Geometry: final body of the model. Coordinates: model frame, mm. Face numbers are marked on the shaded views. A direction names the side the tool comes from. Give positions to 0.01 mm unless a question says otherwise; leave off trailing zeros. Write each loop counter-clockwise with the first axis right and the second up, starting at its lowest first coordinate (ties: lowest second). Pieces come first, ordered by that corner, then holes. Notation, with made-up numbers: (-5, 67) -> (15, 67) arc R28 cw to (15, 86) -> close; hole circle Ø11 at (-20, 48). An arc over 180 degrees is marked (long way). Use CSV: the item, a comma, the result in double quotes. Start each with the question number.
1) Draft query along X for the marked faces 1, 2, 3 and 4. Return one class per face: pulls with the +X half, pulls with the -X half, needs draft (parallel to the pull), parting line crosses it, or undercut.
2) Material intervals for line 1 (Y direction, x = -26, z = 1.9); line 2 (X direction, y = 15.5, z = 6.25); line 3 (Z direction, x = -39, y = -1.5), sorted ascending. Write a range as [from, to].
3) Section D-D (y = -1). Output: boundary loops of the cut face in (x, z).
4) Set-up query: the marked faces 5, 6 and 7. Return all of +Z, -Z, +X, -X, +Y, -Y with unobstructed straight access to the full face (end or side cutting, diameter ignored); none if empty.
5) Contact query for flat-ended pins moving along their axis: P1, Ø3, axis at x = 29, z = 17.5, coming from the +Y side; P2, Ø7, axis at x = 7, y = -15.5, coming from the +Z side; P3, Ø21, axis at x = -44, y = -10.5, coming from the -Z side; P4, Ø2, axis at x = -37, y = 12, coming from the +Z side. Output: stop coordinate, or through.
6) Section C-C (y = -46). Output: boundary loops of the cut face in (x, z).
7) Section B-B (z = 11.25). Output: boundary loops of the cut face in (x, y), plus the area to 3 significant figures.
8) Section A-A (x = -26). Output: boundary loops of the cut face in (y, z), plus the area to 3 significant figures.
```python
from build123d import *

# Parameters (mm, degrees)
CROQUIS1_W              = 116
CROQUIS1_H              = 112
SALIENTE_EXTRUIR1_DEPTH = 3
CROQUIS2_W              = 24
CROQUIS2_H              = 48
SALIENTE_EXTRUIR2_DEPTH = 16
CROQUIS3_W              = 32
CROQUIS3_H              = 17
SALIENTE_EXTRUIR3_DEPTH = 22
VACIADO1_START          = -21.5
VACIADO1_OUTLINE_W      = 27
VACIADO1_OUTLINE_H      = 22.5
VACIADO1_OUTLINE_W_2    = 19
VACIADO1_OUTLINE_H_2    = 14
VACIADO1_DEPTH          = 14.5
VACIADO1_START_2        = -7
VACIADO1_2_OUTLINE_W    = 19
VACIADO1_2_OUTLINE_H    = 14
VACIADO1_2_DEPTH        = 28.5
CROQUIS5_W              = 27
CROQUIS5_H              = 2.5
SALIENTE_EXTRUIR7_DEPTH = 14.5
CORTAR_EXTRUIR1_DEPTH   = 34.5
CROQUIS7_R              = 1.5
CORTAR_EXTRUIR2_DEPTH   = 34.5


# Read off the part's stored shape, not the designer's step: Vaciado1
with BuildPart() as part:
    # Croquis1 → Saliente-Extruir1 (new body)
    with BuildSketch(Plane.XY):
        Rectangle(CROQUIS1_W, CROQUIS1_H)
    extrude(amount=SALIENTE_EXTRUIR1_DEPTH)

    # Croquis2 → Saliente-Extruir2 (add)
    with BuildSketch(Plane.XY.offset(3)):
        with Locations((-40, 0)):
            Rectangle(CROQUIS2_W, CROQUIS2_H)
    extrude(amount=SALIENTE_EXTRUIR2_DEPTH)

    # Croquis3 → Saliente-Extruir3 (add)
    with BuildSketch(Plane.XY.offset(3)):
        with Locations((10, -15.5)):
            Rectangle(CROQUIS3_W, CROQUIS3_H)
    extrude(amount=SALIENTE_EXTRUIR3_DEPTH)

    # Vaciado1 outline → Vaciado1 (cut)
    with BuildSketch(Plane(origin=(0, 0, 0), x_dir=(1, 0, 0), z_dir=(0, 1, 0)).offset(VACIADO1_START)):
        with Locations((10, -13.75)):
            Rectangle(VACIADO1_OUTLINE_W, VACIADO1_OUTLINE_H)
        with Locations((-40, -9.5)):
            Rectangle(VACIADO1_OUTLINE_W_2, VACIADO1_OUTLINE_H_2)
    extrude(amount=VACIADO1_DEPTH, mode=Mode.SUBTRACT)

    # Vaciado1 2 outline → Vaciado1 2 (cut)
    with BuildSketch(Plane(origin=(0, 0, 0), x_dir=(1, 0, 0), z_dir=(0, 1, 0)).offset(VACIADO1_START_2)):
        with Locations((-40, -9.5)):
            Rectangle(VACIADO1_2_OUTLINE_W, VACIADO1_2_OUTLINE_H)
    extrude(amount=VACIADO1_2_DEPTH, mode=Mode.SUBTRACT)

    # Croquis5 → Saliente-Extruir7 (add)
    with BuildSketch(Plane(origin=(0, -21.5, 0), x_dir=(1, 0, 0), z_dir=(0, 1, 0))):
        with Locations((10, -3.75)):
            Rectangle(CROQUIS5_W, CROQUIS5_H)
    extrude(amount=SALIENTE_EXTRUIR7_DEPTH)

    # Croquis6 → Cortar-Extruir1 (cut)
    with BuildSketch(Plane(origin=(26, 0, 0), x_dir=(0, 0, -1), z_dir=(1, 0, 0))):
        Polygon((-25, -7), (-25, -21.5), (-5.5, -7), align=None)
    extrude(amount=-CORTAR_EXTRUIR1_DEPTH, mode=Mode.SUBTRACT)

    # Croquis7 → Cortar-Extruir2 (cut)
    with BuildSketch(Plane.XY.offset(3)):
        with Locations((-26, 46)):
            Circle(CROQUIS7_R)
        with Locations((46, 46)):
            Circle(CROQUIS7_R)
        with Locations((0, -46)):
            Circle(CROQUIS7_R)
    extrude(amount=-CORTAR_EXTRUIR2_DEPTH, mode=Mode.SUBTRACT)


solid = part.part
```
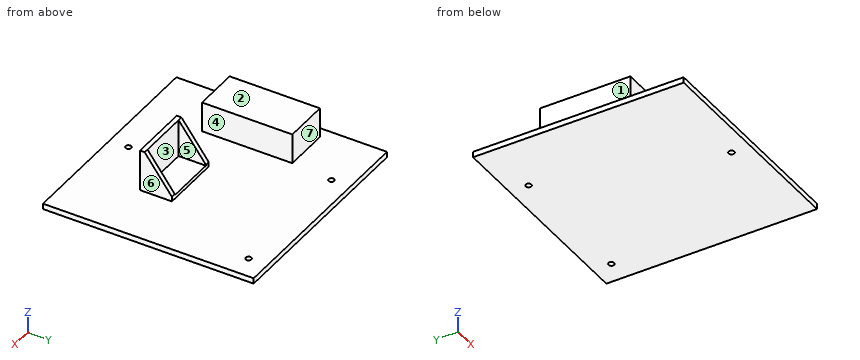
Answers follow:
1,face 1,"pulls with the -X half"
1,face 2,"needs draft"
1,face 3,"undercut"
1,face 4,"undercut"
2,line 1,"y = [-56, 44.5], [47.5, 56]"
2,line 2,"x = [-52, -49.5], [-30.5, -28]"
2,line 3,"z = [0, 2.5], [16.5, 19]"
3,outline,"(-58, 0) -> (58, 0) -> (58, 3) -> (-28, 3) -> (-28, 19) -> (-52, 19) -> (-52, 3) -> (-58, 3) -> close; hole (-49.5, 2.5) -> (-30.5, 2.5) -> (-30.5, 16.5) -> (-49.5, 16.5) -> close"
4,face 5,"+Z, +Y"
4,face 6,"+Z, +X, +Y, -Y"
4,face 7,"+Z, +X, -X, +Y"
5,P1,"passes through"
5,P2,"stops at z = 5"
5,P3,"stops at z = 0"
5,P4,"stops at z = 19"
6,outline,"(-58, 0) -> (-1.5, 0) -> (-1.5, 3) -> (-58, 3) -> close; (1.5, 0) -> (58, 0) -> (58, 3) -> (1.5, 3) -> close"
7,outline,"(-52, -24) -> (-28, -24) -> (-28, 24) -> (-52, 24) -> close; (-6, -24) -> (26, -24) -> (26, -11.28) -> (23.5, -11.28) -> (23.5, -21.5) -> (-3.5, -21.5) -> (-3.5, -11.28) -> (-6, -11.28) -> close; hole (-49.5, -21.5) -> (-30.5, -21.5) -> (-30.5, 21.5) -> (-49.5, 21.5) -> close"
7,area,"466 mm^2"
8,outline,"(-56, 0) -> (44.5, 0) -> (44.5, 3) -> (-56, 3) -> close; (47.5, 0) -> (56, 0) -> (56, 3) -> (47.5, 3) -> close"
8,area,"327 mm^2"
